from build123d import *

# Parameters (mm, degrees)
REVOLUCI_N1_ANGLE     = 180
CROQUIS2_W            = 2
CROQUIS2_H            = 3
CORTAR_EXTRUIR1_DEPTH = 20
CORTAR_EXTRUIR2_DEPTH = 8.865505


with BuildPart() as part:
    # Croquis1 → Revolución1 (revolve)
    with BuildSketch(Plane.XY):
        with BuildLine():
            Line((-49.782166939, -2.382597623), (-32.714919408, -2.382597623))
            Line((-32.714919408, -2.382597623), (-32.714919408, -12.382597623))
            Line((-32.714919408, -12.382597623), (-31.082166939, -12.382597623))
            Line((-31.082166939, -12.382597623), (-31.082166939, -17.382597623))
            Line((-31.082166939, -17.382597623), (-34.282166939, -12.382597623))
            Line((-34.282166939, -12.382597623), (-37.282166939, -12.382597623))
            Line((-37.282166939, -12.382597623), (-37.282166939, -3.882597623))
            Line((-37.282166939, -3.882597623), (-38.282166939, -3.882597623))
            Line((-38.282166939, -3.882597623), (-41.282166939, -3.882597623))
            Line((-41.282166939, -3.882597623), (-51.282166939, -3.882597623))
            Line((-51.282166939, -3.882597623), (-51.282166939, -2.382597623))
            ThreePointArc((-51.282166939, -2.382597623), (-44.838516125, 13.173751563), (-29.282166939, 19.617402377))
            Line((-29.282166939, 19.617402377), (-29.282166939, 18.117402377))
            ThreePointArc((-29.282166939, 18.117402377), (-43.777855954, 12.113091391), (-49.782166939, -2.382597623))
        make_face()
    revolve(axis=Axis((-29.282166939, 18.117402377, 0), (0, 1, 0)), revolution_arc=REVOLUCI_N1_ANGLE)

    # Croquis2 → Cortar-Extruir1 (cut)
    with BuildSketch(Plane(origin=(0, 0, 0), x_dir=(-1, 0, 0), z_dir=(0, 0, -1))):
        with Locations((34.714919408, -9.882597623)):
            Rectangle(CROQUIS2_W, CROQUIS2_H)
        with Locations((34.714919408, -5.882597623)):
            Rectangle(CROQUIS2_W, CROQUIS2_H)
        with Locations((23.84941447, -9.882597623)):
            Rectangle(CROQUIS2_W, CROQUIS2_H)
        with Locations((23.84941447, -5.882597623)):
            Rectangle(CROQUIS2_W, CROQUIS2_H)
    extrude(amount=-CORTAR_EXTRUIR1_DEPTH, mode=Mode.SUBTRACT)

    # Croquis3 → Cortar-Extruir2 (cut)
    with BuildSketch(Plane.ZY.offset(33.714919408)):
        Polygon((6.659632539, -7.382597623), (4.659632539, -7.382597623), (4.659632539, -4.382597623), (9.659632539, -4.382597623), (9.659632539, -7.382597623), align=None)
        Polygon((6.659632539, -11.382597623), (4.659632539, -11.382597623), (4.659632539, -8.382597623), (9.659632539, -8.382597623), (9.659632539, -11.382597623), align=None)
    extrude(amount=-CORTAR_EXTRUIR2_DEPTH, mode=Mode.SUBTRACT)


solid = part.part
CAD build for the part. Positions are in the model's coordinates, mm. A direction names the side the tool comes from. Give positions to 0.01 mm unless a question says otherwise; leave off trailing zeros. Order: outer loops, then holes, each group sorted by start corner. A loop starts at its lowest first (then second) coordinate and runs counter-clockwise, first axis right, second up. Notation, with made-up numbers: (-30, 49.5) - (-13, 49.5) arc R8 cw to (-13, 58.5) - close; hole circle Ø3 at (-33, 2). An arc over 180 degrees is marked (long way). Answer in a Markdown table with one row per item.
1. Saw through at D-D, the plane x = -48. Give the cut face in (y, z).
Data:
| item | result |
|---|---|
| outline | (-3.88, 0) - (-2.38, 0) - (-2.38, 8.36) arc R8.36 cw to (5.98, 0) - (9.18, 0) arc R11.56 ccw to (-2.38, 11.56) - (-3.88, 11.56) - close |
2. Saw through at A-A, the plane x = -42.5. Give the cut face in (y, z).
Data:
| item | result |
|---|---|
| outline | (-3.88, 0) - (-2.38, 0) - (-2.38, 15.67) arc R15.67 cw to (13.29, 0) - (15.2, 0) arc R17.59 ccw to (-2.38, 17.59) - (-3.88, 17.59) - close |
3. Probe probe 1 along Y at (x, z) = (-30, 7.5); probe 2 along Y at (x, z) = (-24, 1); probe 3 along X at (y, z) = (9, 15). List the from-to ranges inside material, lowest first. Write a range as [from, to].
Data:
| item | result |
|---|---|
| probe 1 | y = [-12.38, -11.38], [-8.38, -7.38], [-4.38, -2.38], [16.68, 18.29] |
| probe 2 | y = [-12.38, -11.38], [-8.38, -7.38], [-4.38, -2.38], [17.4, 18.95] |
| probe 3 | x = [-40.66, -37.39], [-21.18, -17.91] |
4. Pull direction Y, two halves, no side cores. Call faces 5 (the flat face through (-29, -12.383, 6)), 6 (the flat face through (-24, -3, 0)), 7 (the flat face through (-33.715, -10, 2)): pulls with the +Y half, pulls with the -Y half, needs draft (parallel to the pull), parting line crosses it, or undercut.
Data:
| item | result |
|---|---|
| face 5 | pulls with the -Y half |
| face 6 | needs draft |
| face 7 | undercut |
5. Flat gauge pins, fed straight in: pin 1 (5 mm diameter, centred on x = -33, z = 18, fed in from -Y); pin 2 (0.9 mm diameter, centred on y = -10, z = 3.5, fed in from -X); pin 3 (6 mm diameter, centred on x = -20, y = 3, fed in from +Z); pin 4 (4 mm diameter, centred on y = -6, z = 9.5, fed in from -X). Where does each tip first touch, or does it go through?
Data:
| item | result |
|---|---|
| pin 1 | stops at y = -3.88 |
| pin 2 | stops at x = -36.68 |
| pin 3 | stops at z = 20.6 |
| pin 4 | passes through |
6. Saw through at C-C, the plane z = 2.5. Count the separate pieces of the cut face and the enclosed holes in it, plus the area to 3 significant figures.
Data:
| item | result |
|---|---|
| separate pieces | 1 |
| enclosed holes | 5 |
| area | 245 mm² |
7. Tool access for faces 1 (the cylindrical face through (-29.46, -8.07, 8)), 2 (the flat face through (-29, -2.383, 8)), 3 (the flat face through (-29, -10, 4.66)), 4 (the flat face through (-22.849, -10, 2)): list every direction of +Z, -Z, +X, -X, +Y, -Y with a clear straight run to the whole face (end or side of a thin tool).
Data:
| item | result |
|---|---|
| face 1 | +Z, -Y |
| face 2 | -Z |
| face 3 | +Z |
| face 4 | +Z, -Z |
